Geometry: final body of the model. Coordinates: model frame, mm. A direction names the side the tool comes from. Coordinates: 2 decimals unless noted, no trailing zeros. Write each loop counter-clockwise with the first axis right and the second up, starting at its lowest first coordinate (ties: lowest second). Pieces come first, ordered by that corner, then holes. Notation, with made-up numbers: (-20, 26.5) -> (-4, 26.5) arc R12 cw to (-4, 45.5) -> close; hole circle Ø2 at (-18.5, -19). An arc over 180 degrees is marked (long way). One line per item, written item: value.
```python
from build123d import *

# Parameters (mm, degrees)
F0_R     = 3.81
F1_DEPTH = 4.7625
F3_D     = 3.556
F4_R     = 3.81


with BuildPart() as f1:
    # F0 (on Top) → F1 (new body)
    with BuildSketch(Plane.XY):
        Polygon((66.738463, 63.5), (-60.261537, 63.5), (-60.261537, -26.4668), (-39.789137, -26.4668), (-39.789137, -45.7708), (-60.261537, -45.7708), (-60.261537, -63.5), (66.738463, -63.5), align=None)
        with Locations((-15.730162, 4.080383)):
            Circle(F0_R, mode=Mode.SUBTRACT)
        with Locations((-20.131484, 14.023047)):
            Circle(F0_R, mode=Mode.SUBTRACT)
        with Locations((-5.651537, 0)):
            Circle(F0_R, mode=Mode.SUBTRACT)
        with Locations((-16.376234, 24.227276)):
            Circle(F0_R, mode=Mode.SUBTRACT)
        with Locations((-6.579748, 28.945015)):
            Circle(F0_R, mode=Mode.SUBTRACT)
        with Locations((5.675161, 5.45465)):
            Circle(F0_R, mode=Mode.SUBTRACT)
        with Locations((8.768908, 15.878513)):
            Circle(F0_R, mode=Mode.SUBTRACT)
        with Locations((3.739601, 25.518755)):
            Circle(F0_R, mode=Mode.SUBTRACT)
    extrude(amount=F1_DEPTH)

    # F3 (through all)
    with Locations(Plane.XY.offset(4.7625)):
        with Locations((-55.308537, 58.547), (61.785463, 58.547), (-55.308537, -58.547), (61.785463, -58.547)):
            Hole(F3_D / 2)

    # F4
    f4_edges = [f1.edges().sort_by_distance(p)[0] for p in [
        (-60.261537, 63.5, 2.38125),
        (-60.261537, -63.5, 2.38125),
        (66.738463, -63.5, 2.38125),
        (66.738463, 63.5, 2.38125),
        (-60.261537, -26.4668, 2.38125),
        (-60.261537, -45.7708, 2.38125),
        (-39.789137, -26.4668, 2.38125),
        (-39.789137, -45.7708, 2.38125),
    ]]
    fillet(f4_edges, radius=F4_R)


solid = f1.part
```
(1) Section A-A (y = -32). Return the cut outline in (x, z), then the cut area to 3 significant figures.
Responses:
outline: (-39.79, 0) -> (66.74, 0) -> (66.74, 4.76) -> (-39.79, 4.76) -> close
area: 507 mm2
(2) Pull-direction query (X, two-part tool) for faces 3 (the flat face through (2, -63.5, 2)), 4 (the cylindrical face through (-54, 59.75, 2.35)), 5 (the cylindrical face through (63.56, 58.63, 2.35)), 6 (the cylindrical face through (-40.935, -27.553, 2.415)); classes: released by +X, released by -X, zero draft, split by the parting line, or undercut.
Responses:
face 3: zero draft
face 4: undercut
face 5: undercut
face 6: released by -X
(3) Line query: line 1 (Y direction, x = 61.5, z = 1.7); line 2 (Y direction, x = -44, z = 1.7); line 3 (X direction, y = 23, z = 2.15). Output: solid intervals per line, ascending. Write a range as [from, to].
Responses:
line 1: y = [-63.5, -60.3], [-56.79, 56.79], [60.3, 63.5]
line 2: y = [-63.5, -45.77], [-26.47, 63.5]
line 3: x = [-60.26, -19.98], [-12.77, 0.88], [6.6, 66.74]
(4) Reachability of faces 1 (the flat face through (66.738, -1, 2)), 2 (the flat face through (-50, -26.467, 2)) from +Z, -Z, +X, -X, +Y, -Y: full face, straight path, thin tool, end or side. Return the list, or none.
Responses:
face 1: +Z, -Z, +X, +Y, -Y
face 2: +Z, -Z, -X
